The listing builds one solid part. Answer for the finished solid, in the listing's coordinates (mm). A direction names the side the tool comes from. Coordinates: 2 decimals unless noted, no trailing zeros. Write each loop counter-clockwise with the first axis right and the second up, starting at its lowest first coordinate (ties: lowest second). Pieces come first, ordered by that corner, then holes.
from build123d import *

# Parameters (mm, degrees)
SKETCH1_R                    = 36
SKETCH1_R_2                  = 1
BASE_FLANGE1_DEPTH           = 3
EDGE_FLANGE1_STRIP_W         = 18
EDGE_FLANGE1_STRIP_H         = 3
EDGE_FLANGE1_STRIP_CUT_DEPTH = 92
EDGE_FLANGE1_DEPTH           = 92
EDGE_FLANGE1_START           = 3
EDGE_FLANGE1_PROFILE_W       = 92
EDGE_FLANGE1_PROFILE_H       = 20
EDGE_FLANGE1_PROFILE_R       = 1
EDGE_FLANGE1_FLAT_DEPTH      = 3
FILLET1_R                    = 2
M3_CLEARANCE_HOLE1_D         = 3.2
M3_CLEARANCE_HOLE1_DEPTH     = 136
M3_CLEARANCE_HOLE1_TIP       = 0.96137699
M5_CLEARANCE_HOLE1_D         = 5.3
M5_CLEARANCE_HOLE1_DEPTH     = 136
M5_CLEARANCE_HOLE1_TIP       = 1.59228064


# Sheet-metal steps are written as plain solids
with BuildPart() as part:
    # Sketch1 → Base-Flange1 (new body)
    with BuildSketch(Plane(origin=(0, 0, 0), x_dir=(1, 0, 0), z_dir=(0, 1, 0))):
        with BuildLine():
            Line((-46, 0), (-46, -55))
            Line((-46, -55), (46, -55))
            Line((46, -55), (46, 0))
            ThreePointArc((46, 0), (0, 46), (-46, 0))
        make_face()
        with Locations(Location((0, 0, 0), (0, 0, 270))):
            Circle(SKETCH1_R, mode=Mode.SUBTRACT)
        with Locations(Location((0, 41.5, 0), (0, 0, 270))):
            Circle(SKETCH1_R_2, mode=Mode.SUBTRACT)
        with Locations(Location((29.344931419, 29.344931419, 0), (0, 0, 270))):
            Circle(SKETCH1_R_2, mode=Mode.SUBTRACT)
        with Locations(Location((41.5, 0, 0), (0, 0, 270))):
            Circle(SKETCH1_R_2, mode=Mode.SUBTRACT)
        with Locations(Location((29.344931419, -29.344931419, 0), (0, 0, 270))):
            Circle(SKETCH1_R_2, mode=Mode.SUBTRACT)
        with Locations(Location((0, -41.5, 0), (0, 0, 270))):
            Circle(SKETCH1_R_2, mode=Mode.SUBTRACT)
        with Locations(Location((-29.344931419, -29.344931419, 0), (0, 0, 270))):
            Circle(SKETCH1_R_2, mode=Mode.SUBTRACT)
        with Locations(Location((-41.5, 0, 0), (0, 0, 270))):
            Circle(SKETCH1_R_2, mode=Mode.SUBTRACT)
        with Locations(Location((-29.344931419, 29.344931419, 0), (0, 0, 270))):
            Circle(SKETCH1_R_2, mode=Mode.SUBTRACT)
    extrude(amount=-BASE_FLANGE1_DEPTH)

    # Edge-Flange1 strip (across the edge) → Edge-Flange1 strip cut (cut)
    with BuildSketch(Plane(origin=(-46, 0, 55), x_dir=(0, 0, -1), z_dir=(1, 0, 0))):
        with Locations((-6, -1.5)):
            Rectangle(EDGE_FLANGE1_STRIP_W, EDGE_FLANGE1_STRIP_H)
    extrude(amount=EDGE_FLANGE1_STRIP_CUT_DEPTH, mode=Mode.SUBTRACT)

    # Edge-Flange1 bend section (across the edge) → Edge-Flange1 (add)
    with BuildSketch(Plane(origin=(-46, 0, 55), x_dir=(0, 0, -1), z_dir=(1, 0, 0))):
        with BuildLine():
            Line((-3, 3), (0, 3))
            ThreePointArc((0, 3), (0.878679656, 0.878679656), (3, 0))
            Line((3, 0), (3, -3))
            ThreePointArc((3, -3), (-1.242640687, -1.242640687), (-3, 3))
        make_face()
    extrude(amount=EDGE_FLANGE1_DEPTH)

    # Edge-Flange1 profile (on flange) → Edge-Flange1 flat (add)
    with BuildSketch(Plane.XY.offset(55).offset(EDGE_FLANGE1_START)):
        with Locations((0, 13)):
            Rectangle(EDGE_FLANGE1_PROFILE_W, EDGE_FLANGE1_PROFILE_H)
        with Locations((-30, 16.8)):
            Circle(EDGE_FLANGE1_PROFILE_R, mode=Mode.SUBTRACT)
        with Locations((30, 16.8)):
            Circle(EDGE_FLANGE1_PROFILE_R, mode=Mode.SUBTRACT)
    extrude(amount=-EDGE_FLANGE1_FLAT_DEPTH)

    # Fillet1
    fillet1_edges = [part.edges().sort_by_distance(p)[0] for p in [
        (-46, 23, 56.5),
        (46, 23, 56.5),
    ]]
    fillet(fillet1_edges, radius=FILLET1_R)

    # M3 Clearance Hole1
    with Locations(Plane(origin=(0, 0, 0), x_dir=(1, 0, 0), z_dir=(0, 1, 0))):
        with Locations((0, 41.5), (29.344931419, 29.344931419), (41.5, 0), (29.344931419, -29.344931419), (0, -41.5), (-29.344931419, -29.344931419), (-41.5, 0), (-29.344931419, 29.344931419)):
            Hole(M3_CLEARANCE_HOLE1_D / 2, depth=M3_CLEARANCE_HOLE1_DEPTH)
            with Locations((0, 0, -(M3_CLEARANCE_HOLE1_DEPTH + M3_CLEARANCE_HOLE1_TIP / 2))):  # 118° drill point
                Cone(0, M3_CLEARANCE_HOLE1_D / 2, M3_CLEARANCE_HOLE1_TIP, mode=Mode.SUBTRACT)

    # M5 Clearance Hole1
    with Locations(Plane.XY.offset(58)):
        with Locations((30, 16.8), (-30, 16.8)):
            Hole(M5_CLEARANCE_HOLE1_D / 2, depth=M5_CLEARANCE_HOLE1_DEPTH)
            with Locations((0, 0, -(M5_CLEARANCE_HOLE1_DEPTH + M5_CLEARANCE_HOLE1_TIP / 2))):  # 118° drill point
                Cone(0, M5_CLEARANCE_HOLE1_D / 2, M5_CLEARANCE_HOLE1_TIP, mode=Mode.SUBTRACT)


solid = part.part
Q1. The part is cut by section B-B, the plane x = 0. Write down the section's boundary in (y, z), then the cut area to 3 significant figures.
Answers below:
outline: (-3, -46) - (0, -46) - (0, -43.1) - (-3, -43.1) - close; (-3, -39.9) - (0, -39.9) - (0, -36) - (-3, -36) - close; (-3, 36) - (0, 36) - (0, 39.9) - (-3, 39.9) - close; (-3, 43.1) - (0, 43.1) - (0, 52) arc R3 cw to (3, 55) - (23, 55) - (23, 58) - (3, 58) arc R6 ccw to (-3, 52) - close
area: 140 mm2
Q2. Determine the mould class of faces 1 (the face through (-27.897, 15.188, 56.479)), 2 (the face through (46, -1, 36)), 3 (the face through (-1, 23, 57)) for opening direction Y: released by +Y, released by -Y, zero draft, split by the parting line, or undercut.
Answers below:
face 1: undercut
face 2: zero draft
face 3: released by +Y
Q3. Find the intervals of material crossed by probe 1 along Z at (x, y) = (24, 15.75); probe 2 along Y at (x, z) = (33, -29); probe 3 along X at (y, z) = (-1.5, 29), in increasing order.
Answers below:
probe 1: z = 55 to 58
probe 2: y = -3 to 0
probe 3: x = -46 to -30.91, -27.78 to -21.33, 21.33 to 27.78, 30.91 to 46
Q4. The part is cut by section A-A, the plane y = 16.8. Write down the section's boundary in (x, z), then the cut area to 3 significant figures.
Answers below:
outline: (-46, 55) - (-32.65, 55) - (-32.65, 58) - (-46, 58) - close; (-27.35, 55) - (27.35, 55) - (27.35, 58) - (-27.35, 58) - close; (32.65, 55) - (46, 55) - (46, 58) - (32.65, 58) - close
area: 244 mm2
Q5. Given pin 1 (3 mm diameter, centred on x = 0, z = -41.5, fed in from -Y); pin 2 (5 mm diameter, centred on x = 41.5, z = 0, fed in from +Y); pin 3 (12 mm diameter, centred on x = 20.5, z = 47.5, fed in from +Y); pin 4 (5 mm diameter, centred on y = 0.5, z = -28.5, fed in from -X), each flat-ended and moving along its own axis, determine where each tip first touches the part or whether it passes through.
Answers below:
pin 1: passes through
pin 2: stops at y = 0
pin 3: stops at y = 0.4
pin 4: stops at x = -37.91
Q6. The part is cut by section C-C, the plane z = 41.5. Write down the section's boundary in (x, y), then the cut area to 3 significant figures.
Answers below:
outline: (-46, -3) - (-1.6, -3) - (-1.6, 0) - (-46, 0) - close; (1.6, -3) - (46, -3) - (46, 0) - (1.6, 0) - close
area: 266 mm2
Q7. Which of the six approach directions +Z, -Z, +X, -X, +Y, -Y give full straight-line access (tool end or side, diameter ignored) to faces 4 (the face through (-11, 0, 35)), 5 (the face through (-46, -1, 36))?
Answers below:
face 4: -Z, +X, -X, +Y
face 5: +Z, -Z, -X, +Y, -Y
Q8. The part is cut by section D-D, the plane x = -22. Write down the section's boundary in (y, z).
Answers below:
outline: (-3, -40.4) - (0, -40.4) - (0, -28.5) - (-3, -28.5) - close; (-3, 28.5) - (0, 28.5) - (0, 52) arc R3 cw to (3, 55) - (23, 55) - (23, 58) - (3, 58) arc R6 ccw to (-3, 52) - close
